Part model, mm, in its own coordinate system. Face numbers are marked on the shaded views. A direction names the side the tool comes from. Round coordinates to 2 decimals unless told otherwise and drop trailing zeros. Write each loop counter-clockwise with the first axis right and the second up, starting at its lowest first coordinate (ties: lowest second). Pieces come first, ordered by that corner, then holes.
1) Which spindle directions (+Z, -Z, +X, -X, +Y, -Y) get a long thin tool onto all of the face, cutting with end or side? Do the marked faces 1, 2 and 3. Say none if no direction does.
2) Flat gauge pins, fed straight in: pin 1 (1.5 mm diameter, centred on x = 8, z = 3, fed in from +Y); pin 2 (1.5 mm diameter, centred on x = 3, z = 1.5, fed in from +Y); pin 3 (5 mm diameter, centred on x = 6.5, z = 1, fed in from +Y). Where does each tip first touch, or does it go through?
3) Saw through at A-A on z = 3.75. Write the cut outline in (x, y).
4) Drill centre lines: L1, parallel to X at y = 1.25, z = 3; L2, parallel to Z at x = 2.25, y = -1.5; L3, parallel to Z at x = 2.75, y = -0.5. Where is each one in solid material? Low to high.
5) Saw through at C-C on x = 6.25. Write the cut outline in (y, z), and give its area (3 significant figures).
6) Pull direction Y, two halves, no side cores. Call the marked faces 4, 5, 6 and 7: +Y half, -Y half, draft (parallel to the pull), parting line (faces both ways), or undercut.
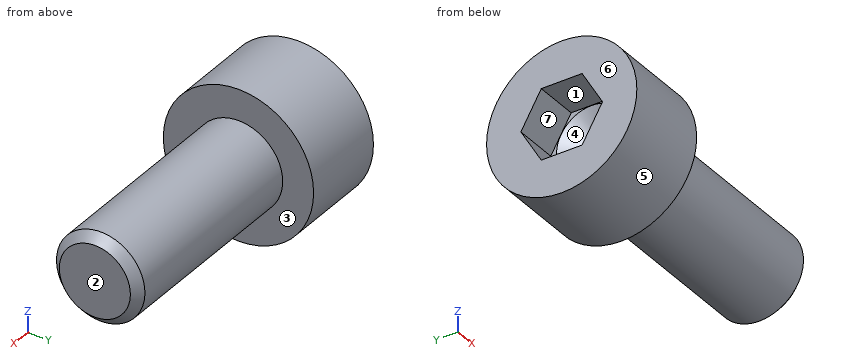
```python
from build123d import *

# Parameters (mm, degrees)
SKETCH1_W           = 5
SKETCH1_H           = 4.25
SKETCH2_R           = 2.5
BOSS_EXTRUDE1_DEPTH = 12
CUT_EXTRUDE1_DEPTH  = 2.5
CHAMFER1_SIZE       = 0.4905


with BuildPart() as part:
    # Sketch1 → Revolve1 (revolve)
    with BuildSketch(Plane(origin=(0, 0, 0), x_dir=(-1, 0, 0), z_dir=(0, 0, -1)), mode=Mode.PRIVATE) as revolve1_sk:
        with Locations((2.5, 2.125)):
            Rectangle(SKETCH1_W, SKETCH1_H)
    revolve(revolve1_sk.sketch.rotate(Axis((0, 0, 0), (-1, 0, 0)), 270), axis=Axis((0, 0, 0), (-1, 0, 0)))

    # Sketch2 → Boss-Extrude1 (add)
    with BuildSketch(Plane(origin=(0, 0, 0), x_dir=(0, 0, -1), z_dir=(1, 0, 0))):
        Circle(SKETCH2_R)
    extrude(amount=BOSS_EXTRUDE1_DEPTH)

    # Sketch3 → Cut-Extrude1 (cut)
    with BuildSketch(Plane.ZY.offset(5)):
        Polygon((2, 1.154700538), (0, 2.309401077), (-2, 1.154700538), (-2, -1.154700538), (0, -2.309401077), (2, -1.154700538), align=None)
    extrude(amount=-CUT_EXTRUDE1_DEPTH, mode=Mode.SUBTRACT)

    # Sketch4 → Cut-Revolve1 (revolve, cut)
    with BuildSketch(Plane.XY, mode=Mode.PRIVATE) as cut_revolve1_sk:
        Polygon((-2.5, 1.99), (-2.5, 0), (-1.351072964, 0), align=None)
    revolve(cut_revolve1_sk.sketch.rotate(Axis((-2.500025, 0, 0), (1, 0, 0)), 90), axis=Axis((-2.500025, 0, 0), (1, 0, 0)), mode=Mode.SUBTRACT)

    # Chamfer1
    chamfer1_edges = [part.edges().sort_by_distance(p)[0] for p in [
        (12, 0, 2.5),
    ]]
    chamfer(chamfer1_edges, length=CHAMFER1_SIZE)


solid = part.part
```
Completed:
1. face 1: -X
1. face 2: +Z, -Z, +X, +Y, -Y
1. face 3: +X
2. pin 1: stops at y = 1.09
2. pin 2: stops at y = 2.38
2. pin 3: stops at y = 2.5
3. outline: (-5, -2) - (0, -2) - (0, 2) - (-5, 2) - close
4. L1: x = -5 to 0
4. L2: z = -2 to 2
4. L3: z = -2.45 to 2.45
5. outline: circle Ø5 at (0, 0)
5. area: 19.6 mm2
6. face 4: undercut
6. face 5: parting line
6. face 6: draft
6. face 7: undercut
